Autodesk Inventor part; units mm, degrees
ref_plane "C1_XY" through (0, 0, 0) normal (0, 0, 1) x (1, 0, 0)
ref_plane "C1_YZ" through (0, 0, 0) normal (1, 0, 0) x (0, 1, 0)
ref_plane "C1_ZX" through (0, 0, 0) normal (0, 1, 0) x (0, 0, 1)
sketch "Sketch_64" plane through (0, 0, 0) normal (0, 0, 1) x (1, 0, 0)
  line L0 (-10, -3) -> (-10, -9)
  arc A0 (-10, -9) -> (-9, -10) centre (-9, -9) ccw
  line L1 (-9, -10) -> (9, -10)
  arc A1 (9, -10) -> (10, -9) centre (9, -9) ccw
  line L2 (10, -9) -> (10, 9)
  arc A2 (10, 9) -> (9, 10) centre (9, 9) ccw
  line L3 (9, 10) -> (3, 10)
  line L4 (3, 10) -> (3, 8)
  line L5 (3, 8) -> (6, 8)
  line L6 (6, 8) -> (6, 7.0607)
  line L7 (6, 7.0607) -> (2.9393, 4)
  line L8 (2.9393, 4) -> (0.5196, 4)
  line L9 (0.5196, 4) -> (0, 3.7)
  line L10 (0, 3.7) -> (-0.5196, 4)
  line L11 (-0.5196, 4) -> (-2.9393, 4)
  line L12 (-2.9393, 4) -> (-6, 7.0607)
  line L13 (-6, 7.0607) -> (-6, 8)
  line L14 (-6, 8) -> (-3, 8)
  line L15 (-3, 8) -> (-3, 10)
  line L16 (-3, 10) -> (-9, 10)
  arc A3 (-9, 10) -> (-10, 9) centre (-9, 9) ccw
  line L17 (-10, 9) -> (-10, 3)
  line L18 (-10, 3) -> (-8, 3)
  line L19 (-8, 3) -> (-8, 6)
  line L20 (-8, 6) -> (-7.0607, 6)
  line L21 (-7.0607, 6) -> (-4, 2.9393)
  line L22 (-4, 2.9393) -> (-4, 0.5196)
  line L23 (-4, 0.5196) -> (-3.7, 0)
  line L24 (-3.7, 0) -> (-4, -0.5196)
  line L25 (-4, -0.5196) -> (-4, -2.9393)
  line L26 (-4, -2.9393) -> (-7.0607, -6)
  line L27 (-7.0607, -6) -> (-8, -6)
  line L28 (-8, -6) -> (-8, -3)
  line L29 (-8, -3) -> (-10, -3)
  line L30 (-6, -7.2678) -> (-6, -7.5)
  arc A4 (-6, -7.5) -> (-5.5, -8) centre (-5.5, -7.5) ccw
  line L31 (-5.5, -8) -> (7, -8)
  arc A5 (7, -8) -> (8, -7) centre (7, -7) ccw
  line L32 (8, -7) -> (8, 5.5)
  arc A6 (8, 5.5) -> (7.5, 6) centre (7.5, 5.5) ccw
  line L33 (7.5, 6) -> (7.2678, 6)
  arc A7 (7.2678, 6) -> (6.9142, 5.8536) centre (7.2678, 5.5) ccw
  line L34 (6.9142, 5.8536) -> (4.1464, 3.0858)
  arc A8 (4.1464, 3.0858) -> (4, 2.7322) centre (4.5, 2.7322) ccw
  line L35 (4, 2.7322) -> (4, -1)
  arc A9 (1, -4) -> (4, -1) centre (1, -1) ccw
  line L36 (1, -4) -> (-2.7322, -4)
  arc A10 (-2.7322, -4) -> (-3.0858, -4.1464) centre (-2.7322, -4.5) ccw
  line L37 (-3.0858, -4.1464) -> (-5.8536, -6.9142)
  arc A11 (-5.8536, -6.9142) -> (-6, -7.2678) centre (-5.5, -7.2678) ccw
extrude "Extrusion1" add sketch "Sketch_64" along normal mid plane 500
sketch "Sketch2" plane through (0, 0, 250) normal (0, 0, 1) x (-1, 0, 0)
  point P0 (0, 0)
hole "Hole1" at (0, 0, 250) direction (0, 0, -1) diameter 4.2 end through all both
ref_plane "C1_XY" through (0, 0, 0) normal (0, 0, 1) x (1, 0, 0)
ref_plane "C1_YZ" through (0, 0, 0) normal (1, 0, 0) x (0, 1, 0)
ref_plane "C1_ZX" through (0, 0, 0) normal (0, 1, 0) x (0, 0, 1)
thread "Thread1"
thread "Thread2"
properties part number "HFST5-2020-500" material "Aluminum 6061"
The model under review builds one solid part; all positions refer to its coordinate system, in mm. Give positions to 0.01 mm unless a question says otherwise; leave off trailing zeros.
1. For P1, Ø2.5, axis at x = -1.5, z = 2, coming from the +Y side; P2, Ø0.7, axis at y = -1.5, z = 7, coming from the -X side, all flat-tipped, find the tip position at first contact; note any pin that passes through.
2. Add section A-A, the plane z = -40.5. Count the separate pieces of the cut face and the enclosed holes in it, plus the area to 3 significant figures.
3. Wall thickness on L1, parallel to Y at x = 0, z = -95; L2, parallel to X at y = 0, z = -20.5; L3, parallel to X at y = -0.5, z = -150.5: over which ranges is each line inside the solid? List them lowest first.
4. Draft analysis for pull direction X (two halves, no side actions). For faces 1 (the flat face through (10, 0, -4)), 2 (the flat face through (8, -1, -4)), 3 (the flat face through (1, -8, -4)), 4 (the flat face through (0, -10, -4)), state which applies: +X half, -X half, draft (parallel to the pull), parting line (faces both ways), or undercut.
Worked answers:
1. P1: stops at y = 4
1. P2: stops at x = -4
2. separate pieces: 1
2. enclosed holes: 2
2. area: 195 mm2
3. L1: y = -10 to -8, -4 to -2.1, 2.1 to 3.7
3. L2: x = -3.7 to -2.1, 2.1 to 4, 8 to 10
3. L3: x = -3.99 to -2.04, 2.04 to 4, 8 to 10
4. face 1: +X half
4. face 2: undercut
4. face 3: undercut
4. face 4: draft
